```python
from build123d import *

# Parameters (mm, degrees)
AUFSATZ_LINEAR_AUSTRAGEN1_DEPTH = 34
SKIZZE2_R                       = 11
AUFSATZ_LINEAR_AUSTRAGEN2_DEPTH = 2
SKIZZE3_R                       = 2.5
AUFSATZ_LINEAR_AUSTRAGEN3_DEPTH = 22
M3_GEWINDEBOHRUNG1_D            = 2.5
M3_GEWINDEBOHRUNG1_DEPTH        = 8.5
M3_GEWINDEBOHRUNG1_TIP          = 0.751075774


with BuildPart() as part:
    # Skizze1 → Aufsatz-Linear austragen1 (new body)
    with BuildSketch(Plane.XY):
        with BuildLine():
            Line((5, 0), (37.3, 0))
            ThreePointArc((37.3, 0), (40.835533906, 1.464466094), (42.3, 5))
            Line((42.3, 5), (42.3, 37.3))
            ThreePointArc((42.3, 37.3), (40.835533906, 40.835533906), (37.3, 42.3))
            Line((37.3, 42.3), (5, 42.3))
            ThreePointArc((5, 42.3), (1.464466094, 40.835533906), (0, 37.3))
            Line((0, 37.3), (0, 5))
            ThreePointArc((0, 5), (1.464466094, 1.464466094), (5, 0))
        make_face()
    extrude(amount=AUFSATZ_LINEAR_AUSTRAGEN1_DEPTH)

    # Skizze2 → Aufsatz-Linear austragen2 (add)
    with BuildSketch(Plane.XY.offset(34)):
        with Locations(Location((21.15, 21.15, 0), (0, 0, 180))):
            Circle(SKIZZE2_R)
    extrude(amount=AUFSATZ_LINEAR_AUSTRAGEN2_DEPTH)

    # Skizze3 → Aufsatz-Linear austragen3 (add)
    with BuildSketch(Plane.XY.offset(36)):
        with Locations((21.15, 21.15)):
            Circle(SKIZZE3_R)
    extrude(amount=AUFSATZ_LINEAR_AUSTRAGEN3_DEPTH)

    # M3 Gewindebohrung1
    with Locations(Plane(origin=(5.65, 36.65, 34), x_dir=(1, 0, 0), z_dir=(0, 0, 1))):
        with Locations((0, 0), (31, 0), (31, -31), (0, -31)):
            Hole(M3_GEWINDEBOHRUNG1_D / 2, depth=M3_GEWINDEBOHRUNG1_DEPTH)
            with Locations((0, 0, -(M3_GEWINDEBOHRUNG1_DEPTH + M3_GEWINDEBOHRUNG1_TIP / 2))):  # 118° drill point
                Cone(0, M3_GEWINDEBOHRUNG1_D / 2, M3_GEWINDEBOHRUNG1_TIP, mode=Mode.SUBTRACT)


solid = part.part
```
The model under review builds one solid part; all positions refer to its coordinate system, in mm. A direction names the side the tool comes from. Round coordinates to 2 decimals unless told otherwise and drop trailing zeros. Order: outer loops, then holes, each group sorted by start corner. A loop starts at its lowest first (then second) coordinate and runs counter-clockwise, first axis right, second up. Notation, with made-up numbers: (71.25, 72) - (85.25, 72) arc R27 ccw to (85.25, 95) - close; hole circle Ø2 at (7, 83.25). An arc over 180 degrees is marked (long way). Answer in a Markdown table with one row per item.
(1) Take a section at D-D on x = 14.5. Write out the cut boundary in (y, z), plus the area to 3 significant figures.
Result set:
| item | result |
|---|---|
| outline | (0, 0) - (42.3, 0) - (42.3, 34) - (29.91, 34) - (29.91, 36) - (12.39, 36) - (12.39, 34) - (0, 34) - close |
| area | 1,470 mm2 |
(2) Mouldability with a two-part tool opening along X and no side actions: class faces 3 (the face through (29.26, 13.72, 34.99)), 4 (the face through (5.81, 37.89, 29.69)), 5 (the face through (5.77, 36.83, 24.88)), 6 (the face through (42.3, 21, 17)) as released by +X, released by -X, zero draft, split by the parting line, or undercut.
Result set:
| item | result |
|---|---|
| face 3 | split by the parting line |
| face 4 | undercut |
| face 5 | undercut |
| face 6 | released by +X |
(3) Machinability: for faces 1 (the face through (5.92, 4.43, 29.69)), 2 (the face through (40.8, 1.43, 16.76)), which of the approach directions +Z, -Z, +X, -X, +Y, -Y give a long, thin tool a straight path to every point of the face, cutting with its end or side? Answer none if there is none.
Result set:
| item | result |
|---|---|
| face 1 | +Z |
| face 2 | +Z, -Z, +X, -Y |
(4) For line 1 (X direction, y = 36.65, z = 31); line 2 (X direction, y = 5, z = 28.5), list the stretches that pass through material, from the lowest coordinate up. Write a range as from..to.
Result set:
| item | result |
|---|---|
| line 1 | x = 0..4.4, 6.9..35.4, 37.9..42.3 |
| line 2 | x = 0..4.58, 6.72..35.58, 37.72..42.3 |
(5) Clearance check with flat-ended pins moving along their axes: P1, Ø1.5, axis at x = 7, y = 29, coming from the +Z side; P2, Ø12, axis at y = 19.5, z = 48, coming from the -X side; P3, Ø12, axis at x = 17.5, y = 10, coming from the +Z side. State where each tip first meets the part, or that it passes through.
Result set:
| item | result |
|---|---|
| P1 | stops at z = 34 |
| P2 | stops at x = 18.65 |
| P3 | stops at z = 36 |
(6) Take a section at C-C on y = 11. Write out the cut boundary in (x, z), plus the area to 3 significant figures.
Result set:
| item | result |
|---|---|
| outline | (0, 0) - (42.3, 0) - (42.3, 34) - (25.39, 34) - (25.39, 36) - (16.91, 36) - (16.91, 34) - (0, 34) - close |
| area | 1,460 mm2 |
(7) Take a section at A-A on y = 21.15. Write out the cut boundary in (x, z).
Result set:
| item | result |
|---|---|
| outline | (0, 0) - (42.3, 0) - (42.3, 34) - (32.15, 34) - (32.15, 36) - (23.65, 36) - (23.65, 58) - (18.65, 58) - (18.65, 36) - (10.15, 36) - (10.15, 34) - (0, 34) - close |
